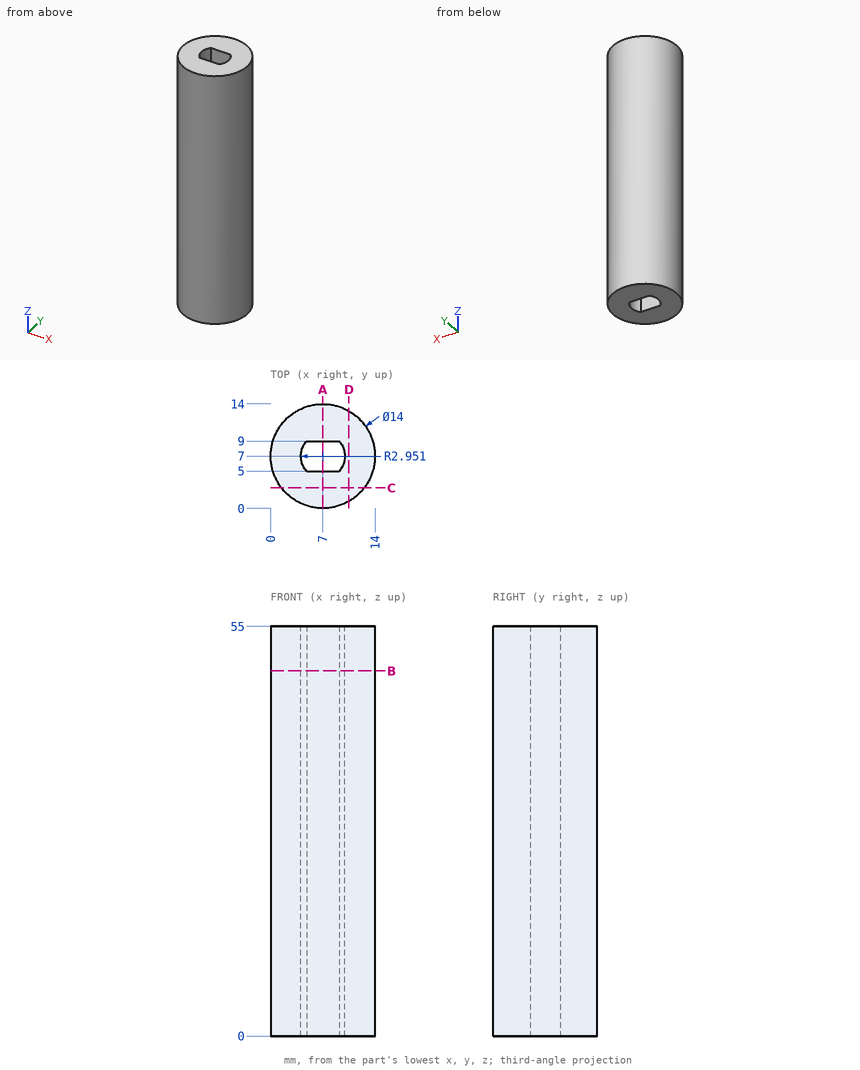
Input: dimensioned drawing with shaded views. Units: mm. Origin: part minimum x, y, z. Coordinates: 2 decimals unless noted, no trailing zeros. Order: outer loops, then holes, each group sorted by start corner. A loop starts at its lowest first (then second) coordinate and runs counter-clockwise, first axis right, second up. Notation, with made-up numbers: M 74.25,35.5 L 79.25,35.5 A28 cw 79.25,61.5 Z; hole C -11.5,10 d10. An arc over 180 degrees is marked long. Write each question's results on one line, items separated by ' | '. Start each with the question number.
Item 1: Cut plane C-C (y = 2.75). Return loops of the section in (x, z).
Item 2: Cut plane D-D (x = 10.5). Return loops of the section in (y, z), and give its area (3 significant figures).
Item 3: Line query: probe 1 along Y at (x, z) = (6.75, 44) (1 decimal); probe 2 along Y at (x, z) = (5.5, 39); probe 3 along X at (y, z) = (6.25, 30.5) (1 decimal). Output: solid intervals per line, ascending.
Item 4: Cut plane A-A (x = 7). Return loops of the section in (y, z).
Item 5: First-contact query: pin 1 Ø1 at (x, z) = (12.5, 46) entering from +Y; pin 2 Ø1.5 at (y, z) = (10.5, 8.5) entering from -X. Flat tips, straight axial feed; report the tip coordinate or a pass-through.
Item 6: Cut plane B-B (z = 49). Return loops of the section in (x, y), and give its area (3 significant figures).
Checked values:
1) outline: M 1.44,0 L 12.56,0 L 12.56,55 L 1.44,55 Z
2) outline: M 0.94,0 L 13.06,0 L 13.06,55 L 0.94,55 Z | area: 667 mm2
3) probe 1: y = 0 to 5, 9 to 14 | probe 2: y = 0.16 to 5, 9 to 13.84 | probe 3: x = 0 to 4.1, 9.9 to 14
4) outline: M 0,0 L 5,0 L 5,55 L 0,55 Z; M 9,0 L 14,0 L 14,55 L 9,55 Z
5) pin 1: stops at y = 11.9 | pin 2: stops at x = 0.56
6) outline: C 7,7 d14; hole M 4.83,5 L 9.17,5 A2.95 ccw 9.17,9 L 4.83,9 A2.95 ccw Z | area: 132 mm2
